```python
from build123d import *

# Parameters (mm, degrees)
SKETCH1_R           = 1.4986
BOSS_EXTRUDE1_DEPTH = 5.159375
SKETCH2_W           = 0.54
SKETCH2_H           = 0.5461
CHAMFER1_SIZE       = 0.254


with BuildPart() as part:
    # Sketch1 → Boss-Extrude1 (new body, symmetric)
    with BuildSketch(Plane.XY):
        Circle(SKETCH1_R)
    extrude(amount=BOSS_EXTRUDE1_DEPTH, both=True)

    # Sketch2 → Cut-Revolve1 (revolve, cut)
    with BuildSketch(Plane(origin=(0, 0, 0), x_dir=(0, 0, -1), z_dir=(1, 0, 0))):
        with Locations((-4.381375, -1.22555)):
            Rectangle(SKETCH2_W, SKETCH2_H)
        with Locations((4.381375, -1.22555)):
            Rectangle(SKETCH2_W, SKETCH2_H)
    revolve(axis=Axis((0, 0, 8.828032455), (0, 0, -1)), mode=Mode.SUBTRACT)

    # Chamfer1
    chamfer1_edges = [part.edges().sort_by_distance(p)[0] for p in [
        (-1.4986, 0, -5.159375),
        (-1.4986, 0, 5.159375),
    ]]
    chamfer(chamfer1_edges, length=CHAMFER1_SIZE)


solid = part.part
```
Geometry check sheet. Reference: the model listing, model coordinates, mm. A direction names the side the tool comes from. Coordinates: 2 decimals unless noted, no trailing zeros. Order: outer loops, then holes, each group sorted by start corner. A loop starts at its lowest first (then second) coordinate and runs counter-clockwise, first axis right, second up.
Q1. Sectioned sample at A-A on y = 0. Record the cut outline in (x, z).
Reply:
outline: (-1.5, -4.91) - (-1.24, -5.16) - (1.24, -5.16) - (1.5, -4.91) - (1.5, -4.65) - (0.95, -4.65) - (0.95, -4.11) - (1.5, -4.11) - (1.5, 4.11) - (0.95, 4.11) - (0.95, 4.65) - (1.5, 4.65) - (1.5, 4.91) - (1.24, 5.16) - (-1.24, 5.16) - (-1.5, 4.91) - (-1.5, 4.65) - (-0.95, 4.65) - (-0.95, 4.11) - (-1.5, 4.11) - (-1.5, -4.11) - (-0.95, -4.11) - (-0.95, -4.65) - (-1.5, -4.65) - close
Q2. Thickness scan on probe 1 along Z at (x, y) = (0.95, -0.65); probe 2 along Z at (x, y) = (-1.3, -0.35); probe 3 along Y at (x, z) = (0.75, 3). Record the ranges inside material, lowest first.
Reply:
probe 1: z = -5.16 to -4.65, -4.11 to 4.11, 4.65 to 5.16
probe 2: z = -5.06 to -4.65, -4.11 to 4.11, 4.65 to 5.06
probe 3: y = -1.3 to 1.3
Q3. Sectioned sample at D-D on y = 1.15. Give the number of separate pieces and of enclosed holes in the cut face, and give its area (3 significant figures).
Reply:
separate pieces: 3
enclosed holes: 0
area: 17.5 mm2
Q4. Sectioned sample at C-C on z = 0.75. Record the cut outline in (x, y), and give its area (3 significant figures).
Reply:
outline: circle Ø3 at (0, 0)
area: 7.06 mm2
Q5. Draft check along Z on faces 3 (the face through (0, 0, 5.159)), 4 (the face through (1.43, 0.45, 0.06)), 5 (the face through (0.58, 0.756, 4.378)). Enter one of: released by +Z, released by -Z, zero draft, split by the parting line, or undercut.
Reply:
face 3: released by +Z
face 4: zero draft
face 5: undercut
Q6. Tool access check on faces 1 (the face through (0.58, 0.756, -4.385)), 2 (the face through (0, 0, -5.159)). Record the directions out of +Z, -Z, +X, -X, +Y, -Y that give a thin tool (end or side, any length) a straight path to the whole face; none if there is none.
Reply:
face 1: none
face 2: -Z, +X, -X, +Y, -Y
